from build123d import *

# Parameters (mm, degrees)
F0_R     = 3.175
F1_DEPTH = 76.2
F5_DEPTH = 3.175


with BuildPart() as f1:
    # F0 (on Front) → F1 (new body, symmetric)
    with BuildSketch(Plane.XZ):
        Circle(F0_R)
    extrude(amount=F1_DEPTH, both=True)

    # F2 (on Top) → F3 (revolve)
    with BuildSketch(Plane.XY):
        Polygon((0, 92.075), (0, 76.2), (3.175, 76.2), align=None)
    revolve(axis=Axis((0, 84.1375, 0), (0, -1, 0)))

    # F4 (on Top) → F5 (join, symmetric)
    with BuildSketch(Plane.XY):
        Polygon((3.175, -76.2), (0, -76.2), (-3.175, -76.2), (-3.175, -83.82), (3.175, -83.82), align=None)
    extrude(amount=F5_DEPTH, both=True)


solid = f1.part
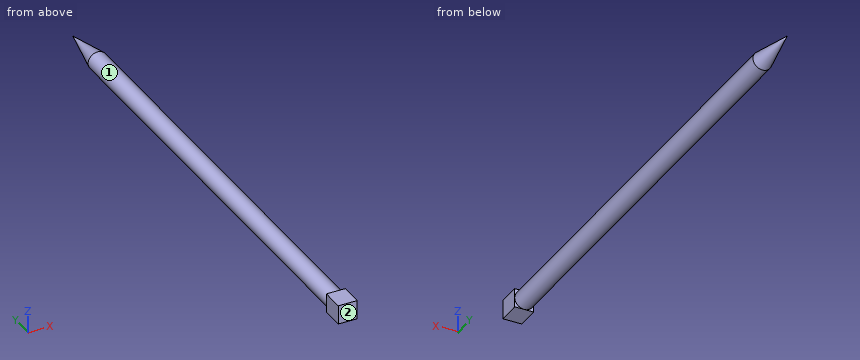
Build history of the part. All positions in model axes, mm. Face numbers are marked on the shaded views. A direction names the side the tool comes from. Round coordinates to 2 decimals unless told otherwise and drop trailing zeros. Write each loop counter-clockwise with the first axis right and the second up, starting at its lowest first coordinate (ties: lowest second). Pieces come first, ordered by that corner, then holes. Notation, with made-up numbers: M -9.5,7.5 L -1.5,7.5 A6 cw -1.5,17.5 Z; hole C 29,-17.5 d6. An arc over 180 degrees is marked long. Answer as a JSON object with one key per item and string values. Group by question number.
(1) Flat gauge pin, fed straight in: pin 1 (1.5 mm diameter, centred on x = 2, y = 57.5, fed in from +Z). Where does the tip first touch, or does it go through?
(2) Drill centre lines: L1, parallel to Y at x = -3, z = 2.5; L2, parallel to Z at x = -0.5, y = 32; L3, parallel to X at y = -72.5, z = -1.75. Where is each one in solid material? Low to high.
(3) Which spindle directions (+Z, -Z, +X, -X, +Y, -Y) get a long thin tool onto all of the face, cutting with end or side? Do the marked faces 1 and 2. Say none if no direction does.
(4) Cut at A-A (y = 69.5). Give the cut face in (x, z) (3 decimals).
Responses:
{
 "1": {"pin 1": "stops at z = 2.92"},
 "2": {"L1": "y = -83.82 to -76.2", "L2": "z = -3.14 to 3.14", "L3": "x = -2.65 to 2.65"},
 "3": {"face 1": "+Y", "face 2": "+Z, -Z, +X, -X, -Y"},
 "4": {"outline": "C 0,0 d6.35"}
}
